Can you work these out from the model? Positions are in its coordinate system, mm. A direction names the side the tool comes from. Round coordinates to 2 decimals unless told otherwise and drop trailing zeros. Write each loop counter-clockwise with the first axis right and the second up, starting at its lowest first coordinate (ties: lowest second). Pieces come first, ordered by that corner, then holes. Notation, with made-up numbers: M 61.5,82.25 L 94.5,82.25 A19 ccw 94.5,106.25 Z; hole C 71,77.25 d9. An arc over 180 degrees is marked long. Answer in a Markdown table with one row per item. Add a question column.
(1) If we mould it in two halves opening along X, with no side actions, what happens to faces 4 (the face through (-9.63, 4.93, -5.67)), 5 (the face through (-1, 0, 12)), 6 (the face through (13.29, 8.75, 17.22))? For each: released by +X, released by -X, zero draft, split by the parting line, or undercut.
(2) For faces 1 (the face through (11.011, 4.659, 11.267)), 2 (the face through (-15, 6, 7)), 3 (the face through (0, 5, 11.176)), which set-ups out of +Z, -Z, +X, -X, +Y, -Y let a thin tool reach every point of the face, with its end or its side?
(3) If I drill on probe 1 along Z at (x, y) = (4.75, 6); probe 2 along Z at (x, y) = (0, 9.5); probe 3 along X at (y, z) = (2.75, -9.5), over which ranges is the centre line in solid material (lowest first)?
(4) Suppose I cut it at D-D, the plane z = 2. Write out the boundary of the cut face in (x, y).
(5) Suppose I cut it at C-C, the plane z = 14.5. Write out the boundary of the cut face in (x, y).
(6) I'm going to push flat-ended pins straight in: pin 1 (3 mm diameter, centred on y = 8, z = 26.5, fed in from +X); pin 2 (3.5 mm diameter, centred on y = 6, z = 14.5, fed in from +X); pin 3 (24.5 mm diameter, centred on x = 6, z = 0, fed in from -Y); pin 4 (4 mm diameter, centred on y = 3, z = 20, fed in from -X). Where does each tip first touch, or does it pass through?
(7) Suppose I cut it at B-B, the plane x = 8.5. Write out the boundary of the cut face in (y, z).
(8) Suppose I cut it at A-A, the plane y = 2. Count the separate pieces of the cut face and the enclosed holes in it, then the cut area to 3 significant figures.
from build123d import *

# Parameters (mm, degrees)
SKETCH1_W           = 30
SKETCH1_H           = 30
BOSS_EXTRUDE1_DEPTH = 12
BOSS_EXTRUDE6_DEPTH = 12
CHAMFER1_SIZE       = 7
CHAMFER1_SIZE2      = 12.124355653
BOSS_EXTRUDE4_DEPTH = 12
SKETCH7_R           = 2.8
CUT_EXTRUDE2_DEPTH  = 15
CHAMFER2_SIZE       = 9
CHAMFER2_SIZE_2     = 14
CHAMFER3_SIZE       = 14
CHAMFER3_SIZE_2     = 9
FILLET2_R           = 20
FILLET3_R           = 1
FILLET4_R           = 1.5
SKETCH10_R          = 1
CUT_EXTRUDE3_DEPTH  = 42.546660516
SKETCH11_R          = 2
CUT_EXTRUDE4_DEPTH  = 42.546660516
SKETCH12_R          = 9
BOSS_EXTRUDE8_DEPTH = 2
SKETCH13_R          = 3.5
CUT_EXTRUDE5_DEPTH  = 8


with BuildPart() as part:
    # Sketch1 → Boss-Extrude1 (new body)
    with BuildSketch(Plane(origin=(0, 0, 0), x_dir=(1, 0, 0), z_dir=(0, 1, 0))):
        Rectangle(SKETCH1_W, SKETCH1_H)
        Polygon((6.452466608, -11.176), (12.904933217, 0), (6.452466608, 11.176), (-6.452466608, 11.176), (-12.904933217, 0), (-6.452466608, -11.176), align=None, mode=Mode.SUBTRACT)
    extrude(amount=BOSS_EXTRUDE1_DEPTH)

    # Sketch8 → Boss-Extrude6 (add)
    with BuildSketch(Plane(origin=(0, 0, 0), x_dir=(1, 0, 0), z_dir=(0, 1, 0))):
        with BuildLine():
            Line((-6, -15), (6, -15))
            Line((6, -15), (6, -29))
            Line((6, -29), (1.7, -29))
            Line((1.7, -29), (1.7, -24))
            ThreePointArc((1.7, -24), (0, -22.3), (-1.7, -24))
            Line((-1.7, -24), (-1.7, -29))
            Line((-1.7, -29), (-6, -29))
            Line((-6, -29), (-6, -15))
        make_face()
    extrude(amount=BOSS_EXTRUDE6_DEPTH)

    # Chamfer1
    chamfer1_edges = [part.edges().sort_by_distance(p)[0] for p in [
        (-15, 6, -15),
        (15, 6, -15),
    ]]
    chamfer1_side = [part.faces().sort_by_distance(p)[0] for p in [
        (0, 6, -15),
    ]]
    chamfer(chamfer1_edges, length=CHAMFER1_SIZE, length2=CHAMFER1_SIZE2, reference=chamfer1_side[0])

    # Sketch6 → Boss-Extrude4 (add)
    with BuildSketch(Plane(origin=(0, 0, 0), x_dir=(1, 0, 0), z_dir=(0, 1, 0))):
        Polygon((-27.223611076, 7.424621202), (-15, -4.798989873), (-15, 2.875644347), (-12.632730187, 6.975875938), (-20.152543264, 14.495689014), align=None)
    extrude(amount=BOSS_EXTRUDE4_DEPTH)

    # Sketch7 → Cut-Extrude2 (cut)
    with BuildSketch(Plane(origin=(-9.899494937, 0, 9.899494937), x_dir=(0.7071067811865438, 0, 0.7071067811865512), z_dir=(-0.7071067811865512, 0, 0.7071067811865438))):
        with Locations((-19.5, 6)):
            Circle(SKETCH7_R)
    extrude(amount=-CUT_EXTRUDE2_DEPTH, mode=Mode.SUBTRACT)

    # Chamfer2
    # the kernel refuses this chamfer: 14, 9 mm, written as the material it adds along each edge
    with BuildSketch(Plane(origin=(6, 0, 15), x_dir=(0.9987204462012896, 0, -0.05057143798130468), z_dir=(0, 1, 0))) as chamfer2_piece_1:
        Polygon((CHAMFER2_SIZE * 0.998720446201, -CHAMFER2_SIZE * 0.0505714379813), (-CHAMFER2_SIZE_2 * 0.0505714379813, -CHAMFER2_SIZE_2 * 0.998720446201), (0, 0), align=None)
    extrude(amount=12)

    # Chamfer3
    # the kernel refuses this chamfer: 14, 9 mm, written as the material it adds along each edge
    with BuildSketch(Plane(origin=(-6, 0, 15), x_dir=(0.020921616646829202, 0, 0.9997811190240007), z_dir=(0, 1, 0))) as chamfer3_piece_1:
        Polygon((CHAMFER3_SIZE * 0.999781119024, -CHAMFER3_SIZE * 0.0209216166468), (-CHAMFER3_SIZE_2 * 0.0209216166468, -CHAMFER3_SIZE_2 * 0.999781119024), (0, 0), align=None)
    extrude(amount=12)

    # Fillet2
    fillet2_edges = [part.edges().sort_by_distance(p)[0] for p in [
        (15, 6, 15),
        (-15, 6, 15),
    ]]
    fillet(fillet2_edges, radius=FILLET2_R)

    # Fillet3
    fillet3_edges = [part.edges().sort_by_distance(p)[0] for p in [
        (-6, 6, 29),
        (-1.7, 6, 29),
        (1.7, 6, 29),
        (6, 6, 29),
    ]]
    fillet(fillet3_edges, radius=FILLET3_R)

    # Fillet4
    fillet4_edges = [part.edges().sort_by_distance(p)[0] for p in [
        (-15, 6, 4.798989873),
        (-12.632730187, 6, -6.975875938),
    ]]
    fillet(fillet4_edges, radius=FILLET4_R)

    # Sketch10 → Cut-Extrude3 (cut, through all)
    with BuildSketch(Plane(origin=(0, 12, 0), x_dir=(1, 0, 0), z_dir=(0, 1, 0))):
        with Locations(Location((0, -14.5, 0), (0, 0, 270))):
            Circle(SKETCH10_R)
    extrude(amount=-CUT_EXTRUDE3_DEPTH, mode=Mode.SUBTRACT)

    # Sketch11 → Cut-Extrude4 (cut, through all)
    with BuildSketch(Plane(origin=(0, 0, 0), x_dir=(0, 0, -1), z_dir=(1, 0, 0))):
        with Locations(Location((-14.5, 6, 0), (0, 0, 180))):
            Circle(SKETCH11_R)
    extrude(amount=CUT_EXTRUDE4_DEPTH, mode=Mode.SUBTRACT)

    # Sketch12 → Boss-Extrude8 (add)
    with BuildSketch(Plane(origin=(0, 12, 0), x_dir=(1, 0, 0), z_dir=(0, 1, 0))):
        Polygon((6.452466608, 11.176), (-6.452466608, 11.176), (-12.904933217, 0), (-6.452466608, -11.176), (6.452466608, -11.176), (12.904933217, 0), align=None)
        with Locations(Location((0, 0, 0), (0, 0, 270))):
            Circle(SKETCH12_R, mode=Mode.SUBTRACT)
    extrude(amount=-BOSS_EXTRUDE8_DEPTH)

    # Sketch13 → Cut-Extrude5 (cut)
    with BuildSketch(Plane(origin=(15, 0, 0), x_dir=(0, 0, -1), z_dir=(1, 0, 0))):
        with Locations((-14.5, 6)):
            Circle(SKETCH13_R)
    extrude(amount=-CUT_EXTRUDE5_DEPTH, mode=Mode.SUBTRACT)


solid = part.part
Calculated:
| question | item | result |
|---|---|---|
| 1 | face 4 | undercut |
| 1 | face 5 | zero draft |
| 1 | face 6 | released by +X |
| 2 | face 1 | +X |
| 2 | face 2 | +Z, -X, +Y, -Y |
| 2 | face 3 | -Y |
| 3 | probe 1 | -15 to -11.18, 11.18 to 12.5, 16.5 to 29 |
| 3 | probe 2 | -15 to -11.18, 11.18 to 13.5, 15.5 to 22.3 |
| 3 | probe 3 | -25.15 to -15.16, -11.18 to -7.42, 7.42 to 11.18 |
| 4 | outline | M -17.8,0 L -11.75,0 L -11.75,10 L -8.77,10 L -8.77,12 L -17.8,12 Z; M 8.77,10 L 11.75,10 L 11.75,0 L 15,0 L 15,12 L 8.77,12 Z |
| 5 | outline | M -14.26,0 L -1,0 L -1,12 L -14.26,12 Z; M 1,0 L 14.26,0 L 14.26,2.5 L 7,2.5 L 7,4 L 1,4 Z; M 1,8 L 7,8 L 7,9.5 L 14.26,9.5 L 14.26,12 L 1,12 Z |
| 6 | pin 1 | x = 8.57 |
| 6 | pin 2 | x = 0 |
| 6 | pin 3 | y = 0 |
| 6 | pin 4 | x = -12.92 |
| 7 | outline | M 0,-14.13 L 12,-14.13 L 12,-2.96 L 10,-2.96 L 10,-7.63 L 0,-7.63 Z; M 0,7.63 L 10,7.63 L 10,2.96 L 12,2.96 L 12,25.11 L 0,25.11 Z; hole C 6,14.5 d7 |
| 8 | separate pieces | 1 |
| 8 | enclosed holes | 2 |
| 8 | area | 776 mm² |
